Check sheet for the modelled part. Datum: model origin and axes. Units: mm. Face numbers are marked on the shaded views. A direction names the side the tool comes from. Round coordinates to 2 decimals unless told otherwise and drop trailing zeros. Loops run counter-clockwise (first coordinate to the right, second up) from the corner with the lowest first, then second, coordinate; pieces in that order, holes last. Notation, with made-up numbers: (36.5, 7) - (47.5, 7) arc R29 ccw to (47.5, 28) - close; hole circle Ø8 at (19, -15). An arc over 180 degrees is marked (long way). Answer in a Markdown table with one row per item. Add a question column.
(1) Access from +Z, -Z, +X, -X, +Y, -Y to the whole of each face (thin tool, end or side, straight path). Record for the marked faces 1, 2, 3, 4 and 5.
(2) Cross-section at B-B on z = 15. Enter the section's corners in (x, y).
(3) Cross-section at C-C on x = 28. Enter the section's corners in (y, z).
(4) Thickness scan on line 1 along X through (y, z) = (-13.5, 22.5); line 2 along Z through (x, y) = (19, -15.5); line 3 along Y through (x, z) = (28, 36.3). Record the ranges inside material, lowest first.
(5) Cross-section at D-D on y = 14. Enter the section's corners in (x, z).
(6) Gauge pin test, flat ends, axial feed: pin 1 (1.5 mm diameter, centred on x = 2, y = -6, fed in from -Z); pin 2 (5 mm diameter, centred on y = -10.5, z = 36, fed in from +X); pin 3 (15 mm diameter, centred on x = 29, y = 8, fed in from +Z); pin 4 (19 mm diameter, centred on x = 28, y = 0, fed in from -Z). Record the tip position at first contact, or that the pin passes through.
(7) Mould release check, pull along Z, two halves, no side actions. Record for the marked faces 6, 7 and 8: +Z half, -Z half, draft (parallel to the pull), parting line (faces both ways), or undercut.
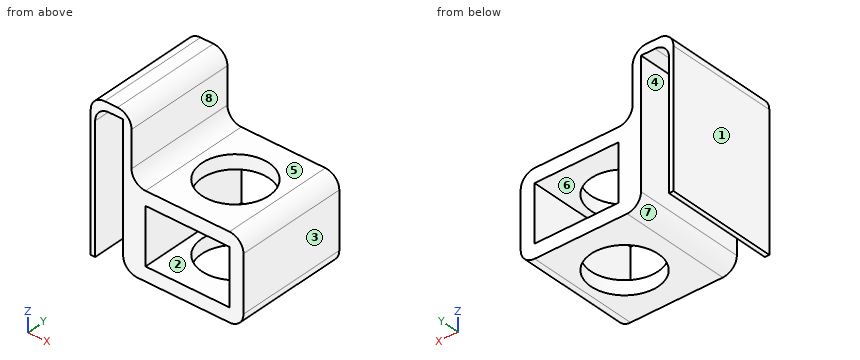
from build123d import *

# Parameters (mm, degrees)
F0_W     = 1.6
F0_H     = 50
F0_W_2   = 40
F0_H_2   = 30
F0_W_3   = 30
F0_H_3   = 20
F1_DEPTH = 20
F3_D     = 24
F4_R     = 5


with BuildPart() as f1:
    # F0 (on Front) → F1 (new body, symmetric)
    with BuildSketch(Plane.XZ):
        with Locations((-5.8, 33.0357266191)):
            Rectangle(F0_W, F0_H)
        Polygon((-6.6, 58.0357266191), (-5, 58.0357266191), (5, 58.0357266191), (5, 61.0357266191), (-6.6, 61.0357266191), align=None)
        Polygon((5, 61.0357266191), (5, 58.0357266191), (5, 8.0357266191), (8, 8.0357266191), (8, 38.0357266191), (8, 61.0357266191), align=None)
        with Locations((28, 23.0357266191)):
            Rectangle(F0_W_2, F0_H_2)
        with Locations((28, 23.0357266191)):
            Rectangle(F0_W_3, F0_H_3, mode=Mode.SUBTRACT)
    extrude(amount=F1_DEPTH, both=True)

    # F3 (through all)
    with Locations(Plane.XY.offset(38.0357266191)):
        with Locations((28, 0)):
            Hole(F3_D / 2)

    # F4
    f4_edges = [f1.edges().sort_by_distance(p)[0] for p in [
        (-5, 0, 58.035727),
        (8, 0, 38.035727),
        (8, 0, 61.035727),
        (-6.6, 0, 61.035727),
        (48, 0, 38.035727),
        (48, 0, 8.035727),
        (5, 0, 8.035727),
    ]]
    fillet(f4_edges, radius=F4_R)


solid = f1.part
Answers:
| question | item | result |
|---|---|---|
| 1 | face 1 | +Z, -Z, -X, +Y, -Y |
| 1 | face 2 | +Y, -Y |
| 1 | face 3 | +Z, -Z, +X, +Y, -Y |
| 1 | face 4 | -Z, +Y, -Y |
| 1 | face 5 | +Z, +X, +Y, -Y |
| 2 | outline | (-6.6, -20) - (-5, -20) - (-5, 20) - (-6.6, 20) - close; (5, -20) - (13, -20) - (13, 20) - (5, 20) - close; (43, -20) - (48, -20) - (48, 20) - (43, 20) - close |
| 3 | outline | (-20, 8.04) - (-12, 8.04) - (-12, 13.04) - (-20, 13.04) - close; (-20, 33.04) - (-12, 33.04) - (-12, 38.04) - (-20, 38.04) - close; (12, 8.04) - (20, 8.04) - (20, 13.04) - (12, 13.04) - close; (12, 33.04) - (20, 33.04) - (20, 38.04) - (12, 38.04) - close |
| 4 | line 1 | x = -6.6 to -5, 5 to 13, 43 to 48 |
| 4 | line 2 | z = 8.04 to 13.04, 33.04 to 38.04 |
| 4 | line 3 | y = -20 to -12, 12 to 20 |
| 5 | outline | (-6.6, 8.04) - (-5, 8.04) - (-5, 53.04) arc R5 cw to (0, 58.04) - (5, 58.04) - (5, 13.04) arc R5 ccw to (10, 8.04) - (43, 8.04) arc R5 ccw to (48, 13.04) - (48, 33.04) arc R5 ccw to (43, 38.04) - (13, 38.04) arc R5 cw to (8, 43.04) - (8, 56.04) arc R5 ccw to (3, 61.04) - (-1.6, 61.04) arc R5 ccw to (-6.6, 56.04) - close; hole (13, 13.04) - (43, 13.04) - (43, 33.04) - (13, 33.04) - close |
| 6 | pin 1 | stops at z = 58.04 |
| 6 | pin 2 | stops at x = 47.98 |
| 6 | pin 3 | stops at z = 38.04 |
| 6 | pin 4 | passes through |
| 7 | face 6 | undercut |
| 7 | face 7 | -Z half |
| 7 | face 8 | draft |
